from build123d import *

# Parameters (mm, degrees)
F0_R     = 1.5
F1_DEPTH = 2


with BuildPart() as f1:
    # F0 (on Top) → F1 (new body)
    with BuildSketch(Plane.XY):
        with BuildLine():
            Line((95, 40), (5, 40))
            ThreePointArc((5, 40), (1.4644660941, 38.5355339059), (0, 35))
            Line((0, 35), (0, 5))
            ThreePointArc((0, 5), (1.4644660941, 1.4644660941), (5, 0))
            Line((5, 0), (95, 0))
            ThreePointArc((95, 0), (98.5355339059, 1.4644660941), (100, 5))
            Line((100, 5), (100, 35))
            ThreePointArc((100, 35), (98.5355339059, 38.5355339059), (95, 40))
        make_face()
        with BuildLine():
            Line((39.9559350041, 24.3510830572), (45.390617828, 24.3510830572))
            Line((45.390617828, 24.3510830572), (45.390617828, 22.8455290317))
            Line((45.390617828, 22.8455290317), (42.4804920591, 22.5012712515))
            add(Edge.make_bspline(
                [(42.4804920591, 22.5012712515), (42.8798310842, 22.0009499442), (43.196548242, 21.1885015829)],
                knots=[0, 0, 0, 1, 1, 1], degree=2))
            add(Edge.make_bspline(
                [(43.196548242, 21.1885015829), (43.5132653998, 20.3760532215), (43.5132653998, 19.3616402958)],
                knots=[0, 0, 0, 1, 1, 1], degree=2))
            add(Edge.make_bspline(
                [(43.5132653998, 19.3616402958), (43.5132653998, 17.0482280127), (41.9342697145, 15.6711968918)],
                knots=[0, 0, 0, 1, 1, 1], degree=2))
            add(Edge.make_bspline(
                [(41.9342697145, 15.6711968918), (40.3552740292, 14.2941657709), (37.6012117874, 14.2941657709)],
                knots=[0, 0, 0, 1, 1, 1], degree=2))
            add(Edge.make_bspline(
                [(37.6012117874, 14.2941657709), (36.8989259157, 14.2941657709), (36.2838520151, 14.4089183643)],
                knots=[0, 0, 0, 1, 1, 1], degree=2))
            add(Edge.make_bspline(
                [(36.2838520151, 14.4089183643), (34.7645276783, 13.6056502104), (34.7645276783, 12.3892727203)],
                knots=[0, 0, 0, 1, 1, 1], degree=2))
            add(Edge.make_bspline(
                [(34.7645276783, 12.3892727203), (34.7645276783, 11.7420680935), (35.2946846599, 11.4345311431)],
                knots=[0, 0, 0, 1, 1, 1], degree=2))
            add(Edge.make_bspline(
                [(35.2946846599, 11.4345311431), (35.8248416414, 11.1269941928), (37.1146607913, 11.1269941928)],
                knots=[0, 0, 0, 1, 1, 1], degree=2))
            Line((37.1146607913, 11.1269941928), (39.8962636556, 11.1269941928))
            add(Edge.make_bspline(
                [(39.8962636556, 11.1269941928), (42.4529514367, 11.1269941928), (43.8208023501, 10.0506148666)],
                knots=[0, 0, 0, 1, 1, 1], degree=2))
            add(Edge.make_bspline(
                [(43.8208023501, 10.0506148666), (45.1886532636, 8.9742355405), (45.1886532636, 6.9224591703)],
                knots=[0, 0, 0, 1, 1, 1], degree=2))
            add(Edge.make_bspline(
                [(45.1886532636, 6.9224591703), (45.1886532636, 4.3106901443), (43.0955659598, 2.940544179)],
                knots=[0, 0, 0, 1, 1, 1], degree=2))
            add(Edge.make_bspline(
                [(43.0955659598, 2.940544179), (41.002478656, 1.5703982137), (36.9861378867, 1.5703982137)],
                knots=[0, 0, 0, 1, 1, 1], degree=2))
            add(Edge.make_bspline(
                [(36.9861378867, 1.5703982137), (33.9015881759, 1.5703982137), (32.2307904159, 2.7179241478)],
                knots=[0, 0, 0, 1, 1, 1], degree=2))
            add(Edge.make_bspline(
                [(32.2307904159, 2.7179241478), (30.5599926558, 3.8654500819), (30.5599926558, 5.9631274894)],
                knots=[0, 0, 0, 1, 1, 1], degree=2))
            add(Edge.make_bspline(
                [(30.5599926558, 5.9631274894), (30.5599926558, 7.3952398552), (31.4780134031, 8.4440785589)],
                knots=[0, 0, 0, 1, 1, 1], degree=2))
            add(Edge.make_bspline(
                [(31.4780134031, 8.4440785589), (32.3960341504, 9.4929172627), (34.0576517029, 9.8647156653)],
                knots=[0, 0, 0, 1, 1, 1], degree=2))
            add(Edge.make_bspline(
                [(34.0576517029, 9.8647156653), (33.4563481135, 10.1355317858), (33.0478288809, 10.7092947528)],
                knots=[0, 0, 0, 1, 1, 1], degree=2))
            add(Edge.make_bspline(
                [(33.0478288809, 10.7092947528), (32.6393096484, 11.2830577198), (32.6393096484, 12.0450149401)],
                knots=[0, 0, 0, 1, 1, 1], degree=2))
            add(Edge.make_bspline(
                [(32.6393096484, 12.0450149401), (32.6393096484, 12.9033643388), (33.098320022, 13.5505689656)],
                knots=[0, 0, 0, 1, 1, 1], degree=2))
            add(Edge.make_bspline(
                [(33.098320022, 13.5505689656), (33.5573303957, 14.1977735924), (34.5487928027, 14.7990771819)],
                knots=[0, 0, 0, 1, 1, 1], degree=2))
            add(Edge.make_bspline(
                [(34.5487928027, 14.7990771819), (33.3278252088, 15.2993984891), (32.5612778849, 16.5043007199)],
                knots=[0, 0, 0, 1, 1, 1], degree=2))
            add(Edge.make_bspline(
                [(32.5612778849, 16.5043007199), (31.7947305609, 17.7092029507), (31.7947305609, 19.2606580136)],
                knots=[0, 0, 0, 1, 1, 1], degree=2))
            add(Edge.make_bspline(
                [(31.7947305609, 19.2606580136), (31.7947305609, 21.8402963134), (33.3438905719, 23.240277953)],
                knots=[0, 0, 0, 1, 1, 1], degree=2))
            add(Edge.make_bspline(
                [(33.3438905719, 23.240277953), (34.8930505829, 24.6402595926), (37.729734692, 24.6402595926)],
                knots=[0, 0, 0, 1, 1, 1], degree=2))
            add(Edge.make_bspline(
                [(37.729734692, 24.6402595926), (38.9644725971, 24.6402595926), (39.9559350041, 24.3510830572)],
                knots=[0, 0, 0, 1, 1, 1], degree=2))
        make_face(mode=Mode.SUBTRACT)
        with BuildLine():
            Line((60.0514091618, 8.6299777602), (58.2842192234, 8.6299777602))
            Line((58.2842192234, 8.6299777602), (57.8114385385, 10.8699483836))
            Line((57.8114385385, 10.8699483836), (57.6966859451, 10.8699483836))
            add(Edge.make_bspline(
                [(57.6966859451, 10.8699483836), (56.5216193886, 9.3919349805), (55.3534379877, 8.8663681027)],
                knots=[0, 0, 0, 1, 1, 1], degree=2))
            add(Edge.make_bspline(
                [(55.3534379877, 8.8663681027), (54.1852565868, 8.3408012249), (52.4318369595, 8.3408012249)],
                knots=[0, 0, 0, 1, 1, 1], degree=2))
            add(Edge.make_bspline(
                [(52.4318369595, 8.3408012249), (50.0954741577, 8.3408012249), (48.7689341779, 9.5479985075)],
                knots=[0, 0, 0, 1, 1, 1], degree=2))
            add(Edge.make_bspline(
                [(48.7689341779, 9.5479985075), (47.4423941981, 10.7551957902), (47.4423941981, 12.9768059986)],
                knots=[0, 0, 0, 1, 1, 1], degree=2))
            add(Edge.make_bspline(
                [(47.4423941981, 12.9768059986), (47.4423941981, 17.7367435731), (55.0573762967, 17.96624876)],
                knots=[0, 0, 0, 1, 1, 1], degree=2))
            Line((55.0573762967, 17.96624876), (57.7242265675, 18.053460731))
            Line((57.7242265675, 18.053460731), (57.7242265675, 19.0311528268))
            add(Edge.make_bspline(
                [(57.7242265675, 19.0311528268), (57.7242265675, 20.8809646325), (56.9301386211, 21.7622645499)],
                knots=[0, 0, 0, 1, 1, 1], degree=2))
            add(Edge.make_bspline(
                [(56.9301386211, 21.7622645499), (56.1360506747, 22.6435644673), (54.3826310475, 22.6435644673)],
                knots=[0, 0, 0, 1, 1, 1], degree=2))
            add(Edge.make_bspline(
                [(54.3826310475, 22.6435644673), (52.4180666483, 22.6435644673), (49.9394106307, 21.4409572884)],
                knots=[0, 0, 0, 1, 1, 1], degree=2))
            Line((49.9394106307, 21.4409572884), (49.2049940329, 23.2632284717))
            add(Edge.make_bspline(
                [(49.2049940329, 23.2632284717), (50.3662902782, 23.8920726836), (51.7502065547, 24.250100775)],
                knots=[0, 0, 0, 1, 1, 1], degree=2))
            add(Edge.make_bspline(
                [(51.7502065547, 24.250100775), (53.1341228312, 24.6081288665), (54.529514367, 24.6081288665)],
                knots=[0, 0, 0, 1, 1, 1], degree=2))
            add(Edge.make_bspline(
                [(54.529514367, 24.6081288665), (57.3386578537, 24.6081288665), (58.6950335078, 23.361915702)],
                knots=[0, 0, 0, 1, 1, 1], degree=2))
            add(Edge.make_bspline(
                [(58.6950335078, 23.361915702), (60.0514091618, 22.1157025376), (60.0514091618, 19.3616402958)],
                knots=[0, 0, 0, 1, 1, 1], degree=2))
            Line((60.0514091618, 19.3616402958), (60.0514091618, 8.6299777602))
        make_face(mode=Mode.SUBTRACT)
        with BuildLine():
            Line((78.0951069494, 8.6299777602), (75.7128431103, 8.6299777602))
            Line((75.7128431103, 8.6299777602), (75.7128431103, 18.80164764))
            add(Edge.make_bspline(
                [(75.7128431103, 18.80164764), (75.7128431103, 20.7203110018), (74.8384283485, 21.6681674233)],
                knots=[0, 0, 0, 1, 1, 1], degree=2))
            add(Edge.make_bspline(
                [(74.8384283485, 21.6681674233), (73.9640135867, 22.6160238449), (72.095841366, 22.6160238449)],
                knots=[0, 0, 0, 1, 1, 1], degree=2))
            add(Edge.make_bspline(
                [(72.095841366, 22.6160238449), (69.6309556596, 22.6160238449), (68.4834297255, 21.2825987095)],
                knots=[0, 0, 0, 1, 1, 1], degree=2))
            add(Edge.make_bspline(
                [(68.4834297255, 21.2825987095), (67.3359037914, 19.9491735741), (67.3359037914, 16.8783941745)],
                knots=[0, 0, 0, 1, 1, 1], degree=2))
            Line((67.3359037914, 16.8783941745), (67.3359037914, 8.6299777602))
            Line((67.3359037914, 8.6299777602), (64.9536399523, 8.6299777602))
            Line((64.9536399523, 8.6299777602), (64.9536399523, 24.3510830572))
            Line((64.9536399523, 24.3510830572), (66.890663729, 24.3510830572))
            Line((66.890663729, 24.3510830572), (67.2762324429, 22.1983244049))
            Line((67.2762324429, 22.1983244049), (67.3909850363, 22.1983244049))
            add(Edge.make_bspline(
                [(67.3909850363, 22.1983244049), (68.1254016341, 23.3596206502), (69.4450564583, 23.9999401214)],
                knots=[0, 0, 0, 1, 1, 1], degree=2))
            add(Edge.make_bspline(
                [(69.4450564583, 23.9999401214), (70.7647112825, 24.6402595926), (72.3850179014, 24.6402595926)],
                knots=[0, 0, 0, 1, 1, 1], degree=2))
            add(Edge.make_bspline(
                [(72.3850179014, 24.6402595926), (75.2262921142, 24.6402595926), (76.6606995318, 23.2701136273)],
                knots=[0, 0, 0, 1, 1, 1], degree=2))
            add(Edge.make_bspline(
                [(76.6606995318, 23.2701136273), (78.0951069494, 21.899967662), (78.0951069494, 18.8842695072)],
                knots=[0, 0, 0, 1, 1, 1], degree=2))
            Line((78.0951069494, 18.8842695072), (78.0951069494, 8.6299777602))
        make_face(mode=Mode.SUBTRACT)
        with Locations((5, 35)):
            Circle(F0_R, mode=Mode.SUBTRACT)
    extrude(amount=F1_DEPTH)


solid = f1.part
For this review, take the finished solid that the model builds, in its own axes (mm). A direction names the side the tool comes from. Round coordinates to 2 decimals unless told otherwise and drop trailing zeros. Write each question's results on one line, items separated by ' | '. Start each with the question number.
1. Add section A-A (z = 1.6). State how many separate pieces and enclosed holes the cut face has, then the cut area to 3 significant figures.
2. Draft analysis for pull direction Y (two halves, no side actions). For faces 3 (the face through (100, 20, 1)), 4 (the face through (49, 0, 1)), 5 (the face through (2, 39, 1)), 6 (the face through (43.956, 22.676, 0.986)), state which applies: pulls with the +Y half, pulls with the -Y half, needs draft (parallel to the pull), parting line crosses it, or undercut.
3. Tool access review of faces 1 (the face through (49, 20, 0)), 2 (the face through (49.577, 22.339, 0.986)): name each direction out of +Z, -Z, +X, -X, +Y, -Y from which nothing blocks a thin tool from reaching the whole face with its end or side.
4. To check wall thickness, follow L1, parallel to Y at x = 40.5, z = 0.45; L2, parallel to Y at x = 5, z = 1.5; L3, parallel to X at y = 14, z = 0.75. State the ranges of each line that lie inside material, in increasing order. Write a range as [from, to].
Output values:
1) separate pieces: 1 | enclosed holes: 4 | area: 3,520 mm^2
2) face 3: needs draft | face 4: pulls with the -Y half | face 5: pulls with the +Y half | face 6: undercut
3) face 1: -Z, +X, -X, +Y, -Y | face 2: +Z, -Z
4) L1: [0, 1.91], [11.11, 14.8], [24.35, 40] | L2: [0, 33.5], [36.5, 40] | L3: [0, 33.49], [35.64, 47.54], [60.05, 64.95], [67.34, 75.71], [78.1, 100]
